Could you check a few things on this model? Use its own coordinates, in mm. Face numbers are marked on the shaded views. Round coordinates to 2 decimals unless told otherwise and drop trailing zeros. Loops run counter-clockwise (first coordinate to the right, second up) from the corner with the lowest first, then second, coordinate; pieces in that order, holes last. Notation, with made-up numbers: (0.25, 5) -> (10.25, 5) arc R17 ccw to (10.25, 14) -> close; hole circle Ø1 at (41.5, 30.25). An arc over 180 degrees is marked (long way). One line per item, written item: value.
```python
from build123d import *

# Parameters (mm, degrees)
F1_DEPTH = 13.97
F2_W     = 12.7
F2_H     = 1.257444
F3_DEPTH = 15.24
F4_W     = 1.27
F4_H     = 1.27
F5_DEPTH = 25.4
F6_W     = 1.27
F6_H     = 1.27
F7_DEPTH = 12.7


with BuildPart() as f1:
    # F0 (on Front) → F1 (new body)
    with BuildSketch(Plane.XZ):
        Polygon((-6.35, 0), (0, 0), (6.35, 0), (6.35, 1.27), (0, 1.27), (-6.35, 1.27), align=None)
    extrude(amount=F1_DEPTH)

    # F2 (on face) → F3 (join)
    with BuildSketch(Plane.XY.offset(1.27)):
        with Locations((0, -0.628722)):
            Rectangle(F2_W, F2_H)
    extrude(amount=F3_DEPTH)

    # F4 (on face) → F5 (join)
    with BuildSketch(Plane(origin=(0, 0, 0), x_dir=(1, 0, 0), z_dir=(0, 0, -1))):
        with Locations((-5.715, 13.335)):
            Rectangle(F4_W, F4_H)
        with Locations((-5.715, 0.635)):
            Rectangle(F4_W, F4_H)
        with Locations((5.715, 0.635)):
            Rectangle(F4_W, F4_H)
        with Locations((5.715, 13.335)):
            Rectangle(F4_W, F4_H)
    extrude(amount=F5_DEPTH)

    # F6 (on face) → F7 (join)
    with BuildSketch(Plane(origin=(0, -12.7, 0), x_dir=(-1, 0, 0), z_dir=(0, 1, 0))):
        with Locations((-5.715, -24.765)):
            Rectangle(F6_W, F6_H)
    extrude(amount=F7_DEPTH)

    # F8: F1 across plane


with BuildPart() as f1_1:
    add(f1.part)
    add(f1.part.mirror(Plane.YZ))


solid = f1_1.part
```
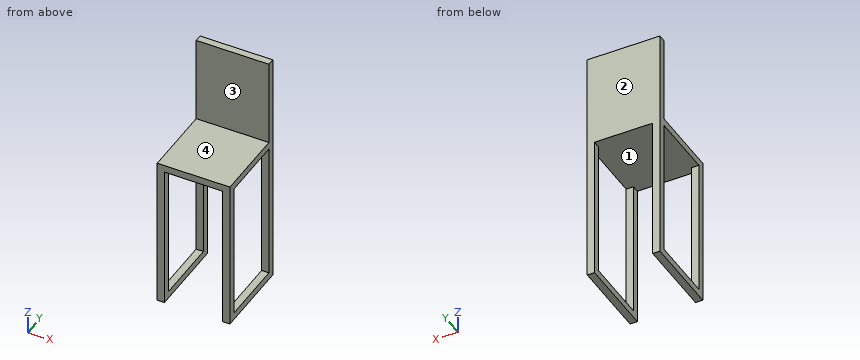
Item 1: If we mould it in two halves opening along Y, with no side actions, what happens to the marked faces 1, 2, 3 and 4? For each: released by +Y, released by -Y, zero draft, split by the parting line, or undercut.
Output:
face 1: undercut
face 2: released by +Y
face 3: released by -Y
face 4: zero draft
Item 2: I need wall thicknesses on line 1 (Z direction, x = 4, y = -12.25); line 2 (Y direction, x = -4, z = 7). Which ranges of each line are inside material? Lowest first, please. Write a range as from..to.
Output:
line 1: z = 0..1.27
line 2: y = -1.26..0
Item 3: If we section it at B-B on y = -5.25: List the corners of the cut face in (x, z) for me.
Output:
outline: (-6.35, -25.4) -> (-5.08, -25.4) -> (-5.08, -24.13) -> (-6.35, -24.13) -> close; (-6.35, 0) -> (6.35, 0) -> (6.35, 1.27) -> (-6.35, 1.27) -> close; (5.08, -25.4) -> (6.35, -25.4) -> (6.35, -24.13) -> (5.08, -24.13) -> close
Item 4: Will these pins go through, and if not, where does the flat tip stop? pin 1 Ø3 at (y, z) = (-11.5, 1.5) entering from +X; pin 2 Ø5 at (x, y) = (0, -2.5) entering from -Z; pin 3 Ø6.5 at (x, y) = (-3, -10.5) entering from +Z; pin 4 Ø3 at (x, z) = (4.5, 4) entering from -Y.
Output:
pin 1: stops at x = 6.35
pin 2: stops at z = 0
pin 3: stops at z = 1.27
pin 4: stops at y = -1.26
Item 5: If we section it at A-A on z = -17: List the corners of the cut face in (x, y) for me, plus the area to 3 significant figures.
Output:
outline: (-6.35, -13.97) -> (-5.08, -13.97) -> (-5.08, -12.7) -> (-6.35, -12.7) -> close; (-6.35, -1.27) -> (-5.08, -1.27) -> (-5.08, 0) -> (-6.35, 0) -> close; (5.08, -13.97) -> (6.35, -13.97) -> (6.35, -12.7) -> (5.08, -12.7) -> close; (5.08, -1.27) -> (6.35, -1.27) -> (6.35, 0) -> (5.08, 0) -> close
area: 6.45 mm²
Item 6: If we section it at C-C on x = 4.5: List the corners of the cut face in (y, z) for me.
Output:
outline: (-13.97, 0) -> (0, 0) -> (0, 16.51) -> (-1.26, 16.51) -> (-1.26, 1.27) -> (-13.97, 1.27) -> close
Item 7: If we section it at D-D on z = 9: List the corners of the cut face in (x, y) for me, plus the area to 3 significant figures.
Output:
outline: (-6.35, -1.26) -> (6.35, -1.26) -> (6.35, 0) -> (-6.35, 0) -> close
area: 16.0 mm²
